The model under review builds one solid part; all positions refer to its coordinate system, in mm. Face numbers are marked on the shaded views. Round coordinates to 2 decimals unless told otherwise and drop trailing zeros. Write each loop counter-clockwise with the first axis right and the second up, starting at its lowest first coordinate (ties: lowest second). Pieces come first, ordered by that corner, then holes. Notation, with made-up numbers: M 82.5,-6 L 118.5,-6 A20 ccw 118.5,-2 Z; hole C 3.25,-11 d8. An arc over 180 degrees is marked long. One line per item, written item: value. Start each with the question number.
1) Mouldability with a two-part tool opening along Z and no side actions: class the marked faces 1 and 2 as +Z half, -Z half, draft (parallel to the pull), parting line (faces both ways), or undercut.
2) For P1, Ø17.5, axis at x = 116.67, z = 10, coming from the +Y side, flat-tipped, find the tip position at first contact; note if it passes through.
3) Take a section at A-A, the plane y = 1.35. Write out the cut boundary in (x, z).
4) Wall thickness on probe 1 along Y at (x, z) = (103, -2.5); probe 2 along Z at (x, y) = (105, 0.4) (3 decimals); probe 3 along Z at (x, y) = (125, 0.2): over which ranges is each line inside the solid? List them lowest first.
Autodesk Fusion 360 part; units mm, degrees
sketch "Sketch1" plane through (0, 0, 0) normal (0, 1, 0) x (1, 0, 0)
  circle A0 centre (116.6706, -10) radius 14.5
  line L0 (137.33, -17.9988) -> (133.9274, 3.8922)
  line L1 (133.9274, 3.8922) -> (113.268, 11.8909)
  line L2 (113.268, 11.8909) -> (96.0112, -2.0012)
  line L3 (96.0112, -2.0012) -> (99.4138, -23.8922)
  line L4 (99.4138, -23.8922) -> (120.0732, -31.8909)
  line L5 (120.0732, -31.8909) -> (137.33, -17.9988)
  point P0 (116.6706, -10)
  dimension "d140" = 29
extrude "Extrude1" add sketch "Sketch1" along normal blind 3
fillet "Fillet1" radius 1 1 edges at (128.7016, 3, 24.9448)
fillet "Fillet2" radius 1 9 edges at (109.2051, 3, 27.6831) (119.7578, 2.7071, 31.7688) (120.0732, 1, 31.8909) (137.33, 1, 17.9988) (137.2781, 2.7071, 17.6646) (135.54, 3, 6.4828) (123.5977, 3, -7.8916) (97.7125, 3, 12.9467) (104.6396, 3, -4.9448)
equation "d140 = buttonOD + 1 mm"
equation "buttonOD = 28 mm"
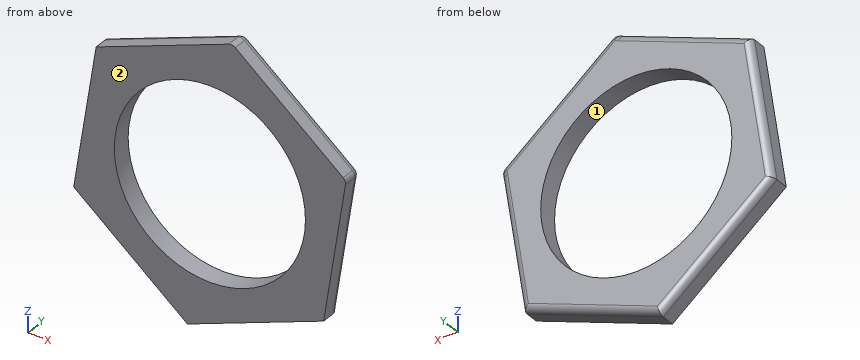
Checked values:
1. face 1: undercut
1. face 2: draft
2. P1: passes through
3. outline: M 96.01,2 L 113.27,-11.89 L 133.93,-3.89 L 137.24,17.43 A1 ccw 136.88,18.36 L 120.52,31.53 A1 ccw 119.53,31.68 L 99.41,23.89 Z; hole C 116.67,10 d29
4. probe 1: y = 0 to 2.99
4. probe 2: z = -5.235 to 1.395, 18.605 to 26.055
4. probe 3: z = -7.35 to -1.87, 21.87 to 27.92
